The figure shows three views and two pictorial views of one solid part (mm, origin at its lowest corner). Answer the questions. A direction names the side the tool comes from. Coordinates: 2 decimals unless noted, no trailing zeros. Write each loop counter-clockwise with the first axis right and the second up, starting at its lowest first coordinate (ties: lowest second). Pieces come first, ordered by that corner, then holes.
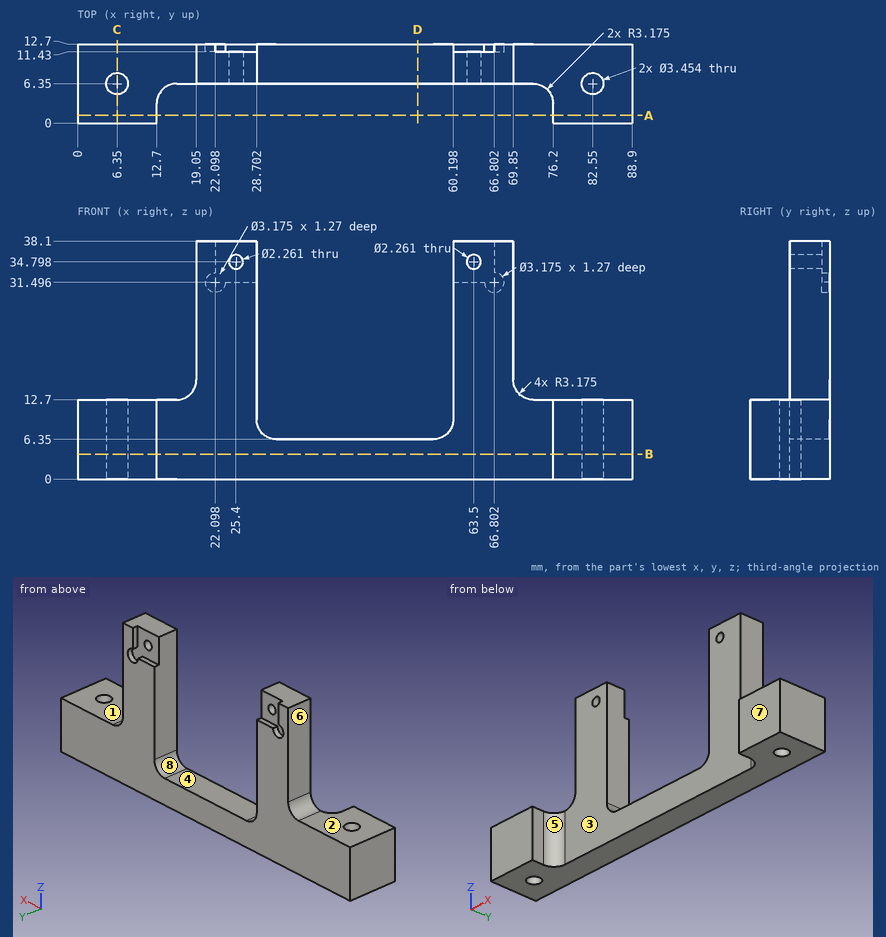
Q1. The part is cut by section A-A, the plane y = 1.25. Write down the section's boundary in (x, z).
Answers below:
outline: (0, 0) - (12.7, 0) - (12.7, 12.7) - (0, 12.7) - close; (76.2, 0) - (88.9, 0) - (88.9, 12.7) - (76.2, 12.7) - close
Q2. Given pin 1 (5 mm diameter, centred on x = 46.5, y = 10.5, fed in from +Z); pin 2 (3 mm diameter, centred on x = 63.5, z = 34.798, fed in from -Y); pin 3 (2.5 mm diameter, centred on x = 66.802, z = 31.496, fed in from +Y), each flat-ended and moving along its own axis, determine where each tip first touches the part or whether it passes through.
Answers below:
pin 1: stops at z = 6.35
pin 2: stops at y = 6.35
pin 3: stops at y = 11.43
Q3. Which of the six approach directions +Z, -Z, +X, -X, +Y, -Y give full straight-line access (tool end or side, diameter ignored) to the marked faces 1, 2, 3 and 4?
Answers below:
face 1: +Z, +X, +Y, -Y
face 2: +Z, -X, +Y, -Y
face 3: +Z, -Z, -Y
face 4: +Z, +Y, -Y
Q4. The part is cut by section D-D, the plane x = 54.5. Write down the section's boundary in (y, z).
Answers below:
outline: (6.35, 0) - (12.7, 0) - (12.7, 6.35) - (6.35, 6.35) - close
Q5. The part is cut by section B-B, the plane z = 4. State how many separate pieces and enclosed holes the cut face has.
Answers below:
separate pieces: 1
enclosed holes: 2
Q6. Find the intervals of material crossed by probe 1 along X at (y, z) = (3, 11); probe 2 along Y at (x, z) = (6.5, 8); probe 3 along X at (y, z) = (7.5, 17), in increasing order.
Answers below:
probe 1: x = 0 to 12.7, 76.2 to 88.9
probe 2: y = 0 to 4.63, 8.07 to 12.7
probe 3: x = 19.05 to 28.7, 60.2 to 69.85
Q7. Determine the mould class of the marked faces 5, 6, 7 and 8 for opening direction X: released by +X, released by -X, zero draft, split by the parting line, or undercut.
Answers below:
face 5: undercut
face 6: released by -X
face 7: zero draft
face 8: undercut
Q8. The part is cut by section C-C, the plane x = 6.35. Write down the section's boundary in (y, z), then the cut area to 3 significant figures.
Answers below:
outline: (0, 0) - (4.62, 0) - (4.62, 12.7) - (0, 12.7) - close; (8.08, 0) - (12.7, 0) - (12.7, 12.7) - (8.08, 12.7) - close
area: 117 mm2
